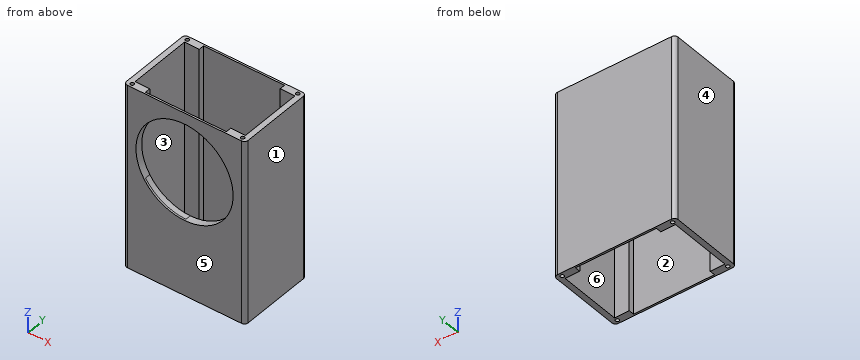
from build123d import *

# Parameters (mm, degrees)
BOSS_EXTRUDE3_DEPTH   = 250
BOSS_EXTRUDE3_2_DEPTH = 250
FILLET1_R             = 5
FILLET2_R             = 5
SKETCH7_R             = 66
CUT_EXTRUDE1_DEPTH    = 10
SKETCH9_R             = 70
SKETCH9_R_2           = 66
BOSS_EXTRUDE4_DEPTH   = 8
SKETCH14_R            = 2.5
CUT_EXTRUDE2_DEPTH    = 12
CUT_EXTRUDE3_START    = -12
SKETCH15_R            = 2.5
CUT_EXTRUDE3_DEPTH    = 12
SKETCH17_W            = 7.5
SKETCH17_H            = 250
BOSS_EXTRUDE5_DEPTH   = 46


with BuildPart() as part:
    # Sketch4 → Boss-Extrude3 (new body)
    with BuildSketch(Plane.XY):
        Polygon((130, 93.5), (130, 86), (150, 86), (150, 66), (155, 66), (157.5, 66), (157.5, 96), (-7.5, 96), (-7.5, 66), (-5, 66), (0, 66), (0, 86), (20, 86), (20, 93.5), align=None)
    extrude(amount=-BOSS_EXTRUDE3_DEPTH)

    # Fillet1
    fillet1_edges = [part.edges().sort_by_distance(p)[0] for p in [
        (-7.5, 96, -125),
        (157.5, 96, -125),
    ]]
    fillet(fillet1_edges, radius=FILLET1_R)


with BuildPart() as body_2:
    # Sketch4 → Boss-Extrude3 2 (new body)
    with BuildSketch(Plane.XY):
        Polygon((155, 20), (150, 20), (150, 0), (130, 0), (130, -7.5), (20, -7.5), (20, 0), (0, 0), (0, 20), (-5, 20), (-7.5, 20), (-7.5, 0), (-7.5, -10), (157.5, -10), (157.5, 20), align=None)
    extrude(amount=-BOSS_EXTRUDE3_2_DEPTH)

    # Fillet2
    fillet2_edges = [body_2.edges().sort_by_distance(p)[0] for p in [
        (157.5, -10, -125),
        (-7.5, -10, -125),
    ]]
    fillet(fillet2_edges, radius=FILLET2_R)

    # Sketch7 → Cut-Extrude1 (cut)
    with BuildSketch(Plane(origin=(0, 0, 0), x_dir=(-1, 0, 0), z_dir=(0, -1, 0))):
        with Locations(Location((-75, 81, 0), (0, 0, 326.442690238))):
            Circle(SKETCH7_R)
    extrude(amount=CUT_EXTRUDE1_DEPTH, mode=Mode.SUBTRACT)

    # Sketch9 → Boss-Extrude4 (add)
    with BuildSketch(Plane.XZ):
        with Locations((75, -81)):
            Circle(SKETCH9_R)
        with Locations(Location((75, -81, 0), (0, 0, 270))):
            Circle(SKETCH9_R_2, mode=Mode.SUBTRACT)
    extrude(amount=BOSS_EXTRUDE4_DEPTH)


with BuildPart() as cut_extrude2_tool:
    # Sketch14 → Cut-Extrude2 (new body)
    with BuildSketch(Plane(origin=(0, 0, -250), x_dir=(-1, 0, 0), z_dir=(0, 0, -1))):
        with Locations((0, 91)):
            Circle(SKETCH14_R)
        with Locations(Location((-150, 91, 0), (0, 0, 180))):
            Circle(SKETCH14_R)
        with Locations(Location((0, -5, 0), (0, 0, 180))):
            Circle(SKETCH14_R)
        with Locations((-150, -5)):
            Circle(SKETCH14_R)
    extrude(amount=-CUT_EXTRUDE2_DEPTH)


with BuildPart() as part_1:
    add(part.part)

    # Cut-Extrude2: cut by cut_extrude2_tool
    add(cut_extrude2_tool.part, mode=Mode.SUBTRACT)


with BuildPart() as body_2_1:
    add(body_2.part)

    # Cut-Extrude2: cut by cut_extrude2_tool
    add(cut_extrude2_tool.part, mode=Mode.SUBTRACT)


with BuildPart() as cut_extrude3_tool:
    # Sketch15 → Cut-Extrude3 (new body)
    with BuildSketch(Plane.XY.offset(CUT_EXTRUDE3_START)):
        with Locations(Location((0, 91, 0), (0, 0, 180))):
            Circle(SKETCH15_R)
        with Locations((150, 91)):
            Circle(SKETCH15_R)
        with Locations(Location((150, -5, 0), (0, 0, 180))):
            Circle(SKETCH15_R)
        with Locations((0, -5)):
            Circle(SKETCH15_R)
    extrude(amount=CUT_EXTRUDE3_DEPTH)


with BuildPart() as part_2:
    add(part_1.part)

    # Cut-Extrude3: cut by cut_extrude3_tool
    add(cut_extrude3_tool.part, mode=Mode.SUBTRACT)



with BuildPart() as body_2_2:
    add(body_2_1.part)

    # Cut-Extrude3: cut by cut_extrude3_tool
    add(cut_extrude3_tool.part, mode=Mode.SUBTRACT)


with BuildPart() as part_3:
    add(part_2.part)

    add(body_2_2.part)  # Boss-Extrude5 merges body 2
    # Sketch17 → Boss-Extrude5 (add)
    with BuildSketch(Plane.XZ.offset(-66)):
        with Locations((-3.75, -125)):
            Rectangle(SKETCH17_W, SKETCH17_H)
        with Locations((153.75, -125)):
            Rectangle(SKETCH17_W, SKETCH17_H)
    extrude(amount=BOSS_EXTRUDE5_DEPTH)


solid = part_3.part
Input: part model. Units: mm. Frame: model coordinates. Face numbers are marked on the shaded views. A direction names the side the tool comes from. Give positions to 0.01 mm unless a question says otherwise; leave off trailing zeros. Write each loop counter-clockwise with the first axis right and the second up, starting at its lowest first coordinate (ties: lowest second). Pieces come first, ordered by that corner, then holes.
Q1. Material intervals for probe 1 along Y at (x, z) = (7, -137); probe 2 along Y at (x, z) = (126.5, -229); probe 3 along X at (y, z) = (79, -98), sorted ascending.
Q2. Section C-C, the plane x = 53. Output: boundary loops of the cut face in (y, z).
Q3. First-contact query: P1, Ø6, axis at x = 60.5, z = -92.5, coming from the -Y side; P2, Ø2.5, axis at x = 150, y = 90.5, coming from the -Z side; P3, Ø4, axis at x = 0, y = -5, coming from the +Z side. Flat tips, straight axial feed; report the tip coordinate or a pass-through.
Q4. Set-up query: the marked faces 1, 2 and 3. Return all of +Z, -Z, +X, -X, +Y, -Y with unobstructed straight access to the full face (end or side cutting, diameter ignored); none if empty.
Q5. Section A-A, the plane y = 63.5. Output: boundary loops of the cut face in (x, z), plus the area to 3 significant figures.
Q6. Section B-B, the plane z = -204. Output: boundary loops of the cut face in (x, y), plus the area to 3 significant figures.
Q7. Pull-direction query (X, two-part tool) for the marked faces 4, 5 and 6; classes: pulls with the +X half, pulls with the -X half, needs draft (parallel to the pull), parting line crosses it, or undercut.
Q8. Section D-D, the plane z = -81. Output: boundary loops of the cut face in (x, y), plus the area to 3 significant figures.
Filled in:
1. probe 1: y = -10 to 0, 86 to 96
1. probe 2: y = -10 to -7.5, 93.5 to 96
1. probe 3: x = -7.5 to 0, 150 to 157.5
2. outline: (-10, -250) - (-7.5, -250) - (-7.5, -147.45) - (0, -147.45) - (0, -143.23) - (-10, -143.23) - close; (-10, -18.77) - (0, -18.77) - (0, -14.55) - (-7.5, -14.55) - (-7.5, 0) - (-10, 0) - close; (93.5, -250) - (96, -250) - (96, 0) - (93.5, 0) - close
3. P1: stops at y = 93.5
3. P2: stops at z = -238
3. P3: stops at z = -12
4. face 1: +Z, -Z, +X, +Y, -Y
4. face 2: -Z
4. face 3: +Z, -Z
5. outline: (-7.5, -250) - (0, -250) - (0, 0) - (-7.5, 0) - close; (150, -250) - (157.5, -250) - (157.5, 0) - (150, 0) - close
5. area: 3,750 mm2
6. outline: (-7.5, -5) arc R5 ccw to (-2.5, -10) - (152.5, -10) arc R5 ccw to (157.5, -5) - (157.5, 91) arc R5 ccw to (152.5, 96) - (-2.5, 96) arc R5 ccw to (-7.5, 91) - close; hole (0, 0) - (20, 0) - (20, -7.5) - (130, -7.5) - (130, 0) - (150, 0) - (150, 86) - (130, 86) - (130, 93.5) - (20, 93.5) - (20, 86) - (0, 86) - close
6. area: 2,920 mm2
7. face 4: pulls with the -X half
7. face 5: needs draft
7. face 6: undercut
8. outline: (-7.5, -5) arc R5 ccw to (-2.5, -10) - (9, -10) - (9, 0) - (0, 0) - (0, 86) - (20, 86) - (20, 93.5) - (130, 93.5) - (130, 86) - (150, 86) - (150, 0) - (141, 0) - (141, -10) - (152.5, -10) arc R5 ccw to (157.5, -5) - (157.5, 91) arc R5 ccw to (152.5, 96) - (-2.5, 96) arc R5 ccw to (-7.5, 91) - close
8. area: 2,420 mm2
